The model under review builds one solid part; all positions refer to its coordinate system, in mm. A direction names the side the tool comes from. Give positions to 0.01 mm unless a question says otherwise; leave off trailing zeros. Loops run counter-clockwise (first coordinate to the right, second up) from the corner with the lowest first, then second, coordinate; pieces in that order, holes last. Notation, with made-up numbers: (-17, 33.5) - (20, 33.5) arc R19 cw to (20, 42.5) - close; hole circle Ø9 at (11.5, 61.25). An arc over 180 degrees is marked (long way). Return JSON: item names as keys, results as strings. Group by question number.
Autodesk Inventor part; units mm, degrees
ref_plane "Work Plane2" through (5, 3, 2) normal (0, 1, 0) x (1, 0, 0)
ref_plane "Work Plane1" through (0, -3, 18) normal (1, 0, 0) x (0, 0, -1)
ref_plane "YZ Plane" through (0, 0, 0) normal (1, 0, 0) x (0, 1, 0)
sketch "Sketch6" plane through (0, 0, 0) normal (0, 0, 1) x (1, 0, 0)
  line L0 (-5, 5) -> (5, 5)
  line L1 (5, 5) -> (5, -5)
  line L2 (5, -5) -> (-5, -5)
  line L3 (-5, -5) -> (-5, 5)
  point P0 (0, 0)
  dimension "d31" = 10
  dimension "d32" = 10
  dimension "d33" = 5
  dimension "d34" = 5
extrude "Extrusion3" add sketch "Sketch6" along normal blind 20
sketch "Sketch7" plane through (0, 0, 20) normal (0, 0, 1) x (1, 0, 0)
  point P0 (0, 0)
  point P1 (0, 0)
hole "Hole4" at (0, 0, 20) direction (0, 0, -1) diameter 3 depth 8
sketch "Sketch8" plane through (-5, 5, 0) normal (0, 1, 0) x (1, 0, 0)
  point P0 (5, 0)
  point P1 (5, -5)
  dimension "d44" = 5
hole "Hole5" at (0, 5, 5) direction (0, -1, 0) diameter 3.1 end through all counterbore diameter 4 counterbore depth 5
sketch "Sketch9" plane through (5, -5, 0) normal (1, 0, 0) x (0, 0, -1)
  line L0 (0, 10) -> (-20, 10) construction
  line L1 (-10, 10) -> (-10, 0) construction
  line L2 (0, 0) -> (-20, 0) construction
  line L3 (0, 0) -> (0, 10)
  line L4 (-10, 8) -> (0, 8)
  line L5 (0, 8) -> (0, 2)
  line L6 (0, 2) -> (-10, 2)
  line L7 (-10, 2) -> (-10, 8)
  line L8 (0, 5) -> (-20, 5)
  line L9 (-20, 10) -> (-20, 0)
  dimension "d52" = 6
extrude "Extrusion4" add sketch "Sketch9" along normal blind 20
ref_plane "Work Plane2" through (5, 3, 2) normal (0, 1, 0) x (1, 0, 0)
sketch "Sketch10" plane through (5, 3, 2) normal (0, 1, 0) x (1, 0, 0)
  line L0 (0, -6) -> (0, 0) construction
  line L1 (0, -3) -> (20, -3) construction
  line L2 (20, -6) -> (20, 0) construction
  point P0 (-5, 2)
  point P1 (15, -3)
  dimension "d56" = 5
hole "Hole6" at (20, 3, 5) direction (0, -1, 0) diameter 3.1 end through all counterbore diameter 4 counterbore depth 3
ref_plane "Work Plane1" through (0, -3, 18) normal (1, 0, 0) x (0, 0, -1)
mirror "Mirror1" about plane through (0, -3, 18) normal (1, 0, 0) of "Extrusion4", "Hole6"
fillet "Fillet3" radius 2 4 edges at (-15, 3, 0) (-15, 3, 10) (-15, -3, 10) (-15, -3, 0)
fillet "Fillet4" radius 2 12 edges at (15, 3, 0) (15, 3, 10) (15, -3, 0) (15, -3, 10) (5, 5, 10) (-5, 5, 10) (-5, -5, 10) (5, -5, 10) (-5, 0, 20) (5, 0, 20) (0, 5, 20) (0, -5, 20)
fillet "Fillet5" radius 2 16 edges at (25, -2.4142, 9.4142) (25, -3, 5) (25, -2.4142, 0.5858) (25, 0, 0) (25, 2.4142, 0.5858) (25, 3, 5) (25, 2.4142, 9.4142) (25, 0, 10) (-25, 0, 10) (-25, -2.4142, 9.4142) (-25, -3, 5) (-25, -2.4142, 0.5858) (-25, 0, 0) (-25, 2.4142, 0.5858) (-25, 3, 5) (-25, 2.4142, 9.4142)
Item 1: Take a section at B-B (z = 14.25). State the section outline as (x, y) points, then the cut area to 3 significant figures.
Item 2: Take a section at D-D (x = 0). State the section outline as (y, z) points, then the cut area to 3 significant figures.
Item 3: Take a section at A-A (x = -20). State the section outline as (y, z) points.
Item 4: For P1, Ø10, axis at x = -8.5, z = 3.5, coming from the -Y side; P2, Ø12, axis at x = -8.5, z = 6, coming from the -Y side; P3, Ø6.5, axis at x = 17, z = 5, coming from the -Y side; P4, Ø0.6, axis at x = -12.5, y = 0, coming from the +Z side, all flat-tipped, find the tip position at first contact; note any pin that passes through.
Item 5: Mouldability with a two-part tool opening along X and no side actions: class faces 4 (the face through (24.4, 2.43, 4.96)), 5 (the face through (0, 2, 3)), 6 (the face through (-0.04, -4.43, 19.4)) as +X half, -X half, draft (parallel to the pull), parting line (faces both ways), or undercut.
Item 6: Take a section at C-C (y = 0.5). State the section outline as (x, z) points, then the cut area to 3 significant figures.
Item 7: For L1, parallel to Z at x = 0, y = 2.05; L2, parallel to X at y = 1.4, z = 5; L3, parallel to Y at x = 0, z = 18, list the stretches that pass through material, from the lowest coordinate up. Write a range as from..to.
Item 8: Tool access review of faces 1 (the face through (14, 0, 10)), 2 (the face through (14, 3, 5)), 3 (the face through (14, -3, 5)): name each direction out of +Z, -Z, +X, -X, +Y, -Y from which nothing blocks a thin tool from reaching the whole face with its end or side.
Check sheet entries:
{
 "1": {"outline": "(-5, -3) arc R2 ccw to (-3, -5) - (3, -5) arc R2 ccw to (5, -3) - (5, 3) arc R2 ccw to (3, 5) - (-3, 5) arc R2 ccw to (-5, 3) - close; hole circle Ø3 at (0, 0)", "area": "89.5 mm^2"},
 "2": {"outline": "(-5, 0) - (5, 0) - (5, 3) - (0, 3) - (0, 3.45) - (-5, 3.45) - close; (-5, 6.55) - (0, 6.55) - (0, 7) - (5, 7) - (5, 18) arc R2 ccw to (3, 20) - (1.5, 20) - (1.5, 12) - (-1.5, 12) - (-1.5, 20) - (-3, 20) arc R2 ccw to (-5, 18) - close", "area": "139 mm^2"},
 "3": {"outline": "(-3, 2) arc R2 ccw to (-1, 0) - (1, 0) arc R2 ccw to (3, 2) - (3, 3) - (0, 3) - (0, 3.45) - (-3, 3.45) - close; (-3, 6.55) - (0, 6.55) - (0, 7) - (3, 7) - (3, 8) arc R2 ccw to (1, 10) - (-1, 10) arc R2 ccw to (-3, 8) - close"},
 "4": {"P1": "stops at y = -4.94", "P2": "stops at y = -5", "P3": "stops at y = -3", "P4": "stops at z = 10"},
 "5": {"face 4": "+X half", "face 5": "undercut", "face 6": "draft"},
 "6": {"outline": "(-25, 2) arc R2 ccw to (-23, 0) - (23, 0) arc R2 ccw to (25, 2) - (25, 8) arc R2 ccw to (23, 10) - (5, 10) - (5, 18) arc R2 ccw to (3, 20) - (1.41, 20) - (1.41, 12) - (-1.41, 12) - (-1.41, 20) - (-3, 20) arc R2 ccw to (-5, 18) - (-5, 10) - (-23, 10) arc R2 ccw to (-25, 8) - close; hole circle Ø4 at (-20, 5); hole circle Ø4 at (0, 5); hole circle Ø4 at (20, 5)", "area": "535 mm^2"},
 "7": {"L1": "z = 0..3, 7..20", "L2": "x = -24.96..-22, -18..-2, 2..18, 22..24.96", "L3": "y = -5..-1.5, 1.5..5"},
 "8": {"face 1": "+Z, +X, +Y, -Y", "face 2": "+Z, -Z, +X, +Y", "face 3": "+Z, -Z, +X, -Y"}
}
